Input: part model. Units: mm. Frame: model coordinates. A direction names the side the tool comes from. Give positions to 0.01 mm unless a question says otherwise; leave off trailing zeros. Loops run counter-clockwise (first coordinate to the right, second up) from the corner with the lowest first, then second, coordinate; pieces in that order, holes last. Notation, with made-up numbers: M 51,-5 L 94,-5 A23 cw 94,4 Z; hole C 51.5,-39 d2. An arc over 180 degrees is marked long. Use CSV: the item, a comma, the result in double quotes. Start each with the question number.
Q1. Section C-C, the plane x = -32.55. Output: boundary loops of the cut face in (y, z), plus the area to 3 significant figures.
Q2. Material intervals for line 1 along Y through (x, z) = (-33.45, 17.3); line 2 along Z through (x, y) = (-33.05, -18.75); line 3 along Z through (x, y) = (-32.35, -19.5), sorted ascending.
Q3. Section D-D, the plane z = 2. Output: boundary loops of the cut face in (x, y).
Q4. Pin query (flat end, axial travel): pin 1 (1.3 mm diameter, centred on x = -30.5, y = -29.5, fed in from +Z); pin 2 (3.5 mm diameter, centred on y = -40, z = 17.3, fed in from +X); pin 3 (1.2 mm diameter, centred on x = -32, z = 7, fed in from +Y). Return the tip coordinate at first contact, or that it passes through.
Q5. Pull-direction query (Y, two-part tool) for faces 1 (the flat face through (-33, -29, 20)), 2 (the flat face through (-32, -42.5, 13)), 3 (the cylindrical face through (-30.51, -17.59, 3.04)), 4 (the flat face through (-32, -15.5, 13)); classes: released by +Y, released by -Y, zero draft, split by the parting line, or undercut.
Q6. Section B-B, the plane y = -40. Output: boundary loops of the cut face in (x, z).
Q7. Section A-A, the plane z = 17.3. Output: boundary loops of the cut face in (x, y).
Q8. Reachability of faces 5 (the flat face through (-32, -18, 8.5)), 6 (the cylindrical face through (-32.087, -41.318, 3.042)), 7 (the flat face through (-32, -37.5, 7)) from +Z, -Z, +X, -X, +Y, -Y: full face, straight path, thin tool, end or side. Return the list, or none.
Autodesk Inventor part; units mm, degrees
ref_plane "작업 평면1" through (-17.0116, -44.6019, 14.5) normal (0, 0, -1) x (0, 1, 0)
ref_plane "YZ Plane" through (0, 0, 0) normal (1, 0, 0) x (0, 1, 0)
ref_plane "XZ Plane" through (0, 0, 0) normal (0, 1, 0) x (-1, 0, 0)
ref_plane "작업 평면1" through (-17.0116, -44.6019, 14.5) normal (0, 0, -1) x (0, 1, 0)
sketch "스케치4" plane through (0, 0, 0) normal (0, 0, 1) x (1, 0, 0)
  arc A0 (-34.0751, 6.2636) -> (-34.5943, 4.5766) centre (-31.5943, 4.5766) ccw
  line L0 (-34.5943, -39.6766) -> (-34.5943, 4.5766)
  arc A1 (-34.5943, -39.6766) -> (-34.0751, -41.3636) centre (-31.5943, -39.6766) ccw
  line L1 (-30.3872, -46.7869) -> (-34.0751, -41.3636)
  arc A2 (-30.3872, -46.7869) -> (-27.9064, -48.1) centre (-27.9064, -45.1) ccw
  line L2 (-1.0822, -48.1) -> (-27.9064, -48.1)
  arc A3 (-1.0822, -48.1) -> (1.3986, -46.7869) centre (-1.0822, -45.1) ccw
  line L3 (5.0865, -41.3636) -> (1.3986, -46.7869)
  arc A4 (5.0865, -41.3636) -> (5.6057, -39.6766) centre (2.6057, -39.6766) ccw
  line L4 (5.6057, 4.5766) -> (5.6057, -39.6766)
  arc A5 (5.6057, 4.5766) -> (5.0865, 6.2636) centre (2.6057, 4.5766) ccw
  line L5 (1.1009, 12.1246) -> (5.0865, 6.2636)
  arc A6 (1.1009, 12.1246) -> (-0.5529, 13) centre (-0.5529, 11) ccw
  line L6 (-6.8443, 13) -> (-0.5529, 13)
  arc A7 (-5.3443, 11.5) -> (-6.8443, 13) centre (-6.8443, 11.5) ccw
  line L7 (-5.3443, 11.5) -> (-5.3443, 10)
  arc A8 (-5.3443, 10) -> (-2.9943, 7.65) centre (-2.9943, 10) ccw
  line L8 (-2.9943, 7.65) -> (-0.9943, 7.65)
  arc A9 (0.0057, 6.65) -> (-0.9943, 7.65) centre (-0.9943, 6.65) ccw
  line L9 (0.0057, 6.65) -> (0.0057, -36.15)
  arc A10 (-0.9943, -37.15) -> (0.0057, -36.15) centre (-0.9943, -36.15) ccw
  line L10 (-0.9943, -37.15) -> (-2.9943, -37.15)
  arc A11 (-2.9943, -37.15) -> (-5.3443, -39.5) centre (-2.9943, -39.5) ccw
  line L11 (-5.3443, -39.5) -> (-5.3443, -41.5)
  arc A12 (-6.3443, -42.5) -> (-5.3443, -41.5) centre (-6.3443, -41.5) ccw
  line L12 (-6.3443, -42.5) -> (-22.6443, -42.5)
  arc A13 (-23.6443, -41.5) -> (-22.6443, -42.5) centre (-22.6443, -41.5) ccw
  line L13 (-23.6443, -41.5) -> (-23.6443, -39.5)
  arc A14 (-23.6443, -39.5) -> (-25.9943, -37.15) centre (-25.9943, -39.5) ccw
  line L14 (-25.9943, -37.15) -> (-27.9943, -37.15)
  arc A15 (-28.9943, -36.15) -> (-27.9943, -37.15) centre (-27.9943, -36.15) ccw
  line L15 (-28.9943, -36.15) -> (-28.9943, 6.65)
  arc A16 (-27.9943, 7.65) -> (-28.9943, 6.65) centre (-27.9943, 6.65) ccw
  line L16 (-27.9943, 7.65) -> (-25.9943, 7.65)
  arc A17 (-25.9943, 7.65) -> (-23.6443, 10) centre (-25.9943, 10) ccw
  line L17 (-23.6443, 10) -> (-23.6443, 11.5)
  arc A18 (-22.1443, 13) -> (-23.6443, 11.5) centre (-22.1443, 11.5) ccw
  line L18 (-28.4357, 13) -> (-22.1443, 13)
  arc A19 (-28.4357, 13) -> (-30.0896, 12.1246) centre (-28.4357, 11) ccw
  line L19 (-34.0751, 6.2636) -> (-30.0896, 12.1246)
  circle A20 centre (2.8057, 4) radius 1.35
  circle A21 centre (2.8057, -18) radius 1.35
  circle A22 centre (-3.4943, -45.3) radius 1.35
  circle A23 centre (-31.7943, 4) radius 1.35
  circle A24 centre (-31.7943, -18) radius 1.35
  circle A25 centre (-25.4943, -45.3) radius 1.35
  circle A26 centre (2.8057, -40) radius 1.35
  circle A27 centre (-31.7943, -40) radius 1.35
  line L20 (-31.7943, -40) -> (-31.7943, -18)
  line L21 (-29.0943, -15.5) -> (-34.4943, -15.5)
  line L22 (-34.4943, -15.5) -> (-34.4943, -42.5)
  line L23 (-34.4943, -42.5) -> (-29.0943, -42.5)
  line L24 (-29.0943, -42.5) -> (-29.0943, -15.5)
  line L25 (-29.0943, -15.5) -> (-34.4943, -42.5) construction
  line L26 (-34.4943, -15.5) -> (-29.0943, -42.5) construction
  point P0 (0, 0)
  point P1 (-31.7943, -29)
  dimension "d10" = 5.4
  dimension "d11" = 27
extrude "돌출4" add sketch "스케치4" against normal blind 6 contours L22 L21 L24 L23 L1 A1 | A1 L1 L23 L22
sketch "스케치5" plane through (0, 0, 0) normal (0, 0, 1) x (1, 0, 0)
  line L0 (-34.4943, -15.5) -> (-34.4943, -42.5)
  line L1 (-34.4943, -42.5) -> (-29.0943, -42.5)
  line L2 (-29.0943, -42.5) -> (-29.0943, -15.5)
  line L3 (-29.0943, -15.5) -> (-34.4943, -15.5)
  circle A0 centre (-31.7943, -40) radius 1.35
  circle A1 centre (-31.7943, -18) radius 1.35
  point P0 (0, 0)
extrude "돌출5" add sketch "스케치5" along normal blind 14.4 contours L3 L2 L1 L0 | A0 | A1
sketch "스케치6" plane through (-34.4943, -42.5, -6) normal (-1, 0, 0) x (0, 0, 1)
  line L0 (25.6, 57) -> (29.1, 57)
  line L1 (25.6, 57) -> (20.5, 51)
  line L2 (20.5, 51) -> (20.5, -2.1)
  line L3 (20.5, -2.1) -> (25.6, -8.1)
  line L4 (25.6, -8.1) -> (55.6, -8.1)
  line L5 (55.6, -8.1) -> (60.7, -2.1)
  line L6 (60.7, -2.1) -> (60.7, 51)
  line L7 (60.7, 51) -> (55.6, 57)
  line L8 (52.1, 57) -> (55.6, 57)
  arc A0 (55.1, 54) -> (52.1, 57) centre (52.1, 54) ccw
  line L9 (55.1, 0.5) -> (55.1, 54)
  arc A1 (52.1, -2.5) -> (55.1, 0.5) centre (52.1, 0.5) ccw
  line L10 (29.1, -2.5) -> (52.1, -2.5)
  arc A2 (26.1, 0.5) -> (29.1, -2.5) centre (29.1, 0.5) ccw
  line L11 (26.1, 54) -> (26.1, 0.5)
  arc A3 (29.1, 57) -> (26.1, 54) centre (29.1, 54) ccw
  circle A4 centre (57.9, 46.5) radius 1.35
  circle A5 centre (57.9, 24.5) radius 1.35
  circle A6 centre (57.9, 2.5) radius 1.35
  circle A7 centre (51.6, -5.3) radius 1.35
  circle A8 centre (23.3, 46.5) radius 1.35
  circle A9 centre (23.3, 24.5) radius 1.35
  circle A10 centre (23.3, 2.5) radius 1.35
  circle A11 centre (29.6, -5.3) radius 1.35
  line L12 (20.4, 27) -> (0, 27)
  line L13 (0, 0) -> (0, 27)
  line L14 (0, 0) -> (20.4, 0)
  line L15 (20.4, 27) -> (20.4, 0)
  line L16 (20.4, 0) -> (20.4, 27)
  line L17 (20.4, 27) -> (26, 27)
  line L18 (26, 27) -> (26, 0)
  line L19 (26, 0) -> (20.4, 0)
  line L20 (25.6959, -1.4327) -> (25.7781, -6.0132)
  line L21 (68.9946, 18.9724) -> (67.812, 18.9512)
  arc A12 (65.7765, 20.915) -> (67.812, 18.9512) centre (67.7762, 20.9508) ccw
  line L22 (65.7765, 20.915) -> (65.7397, 22.9646)
  arc A13 (65.7397, 22.9646) -> (64.7219, 23.9465) centre (64.7399, 22.9467) ccw
  line L23 (64.7219, 23.9465) -> (31.7272, 23.3545)
  arc A14 (31.7272, 23.3545) -> (30.7453, 22.3368) centre (31.7452, 22.3547) ccw
  line L24 (30.7453, 22.3368) -> (30.7821, 20.2871)
  arc A15 (28.8183, 18.2515) -> (30.7821, 20.2871) centre (28.7824, 20.2512) ccw
  line L25 (28.8183, 18.2515) -> (26.8186, 18.2157)
  arc A16 (26.8186, 18.2157) -> (25.8367, 17.1979) centre (26.8366, 17.2158) ccw
  line L26 (25.8367, 17.1979) -> (26.0574, 4.8999)
  arc A17 (26.0574, 4.8999) -> (27.0752, 3.918) centre (27.0572, 4.9178) ccw
  line L27 (27.0752, 3.918) -> (29.0748, 3.9538)
  arc A18 (31.1104, 1.99) -> (29.0748, 3.9538) centre (29.1107, 1.9542) ccw
  line L28 (31.1104, 1.99) -> (31.1472, -0.0596)
  arc A19 (31.1472, -0.0596) -> (32.165, -1.0415) centre (32.147, -0.0417) ccw
  line L29 (32.165, -1.0415) -> (65.1596, -0.4495)
  arc A20 (65.1596, -0.4495) -> (66.1415, 0.5682) centre (65.1417, 0.5503) ccw
  line L30 (66.1415, 0.5682) -> (66.1048, 2.6179)
  arc A21 (68.0686, 4.6535) -> (66.1048, 2.6179) centre (68.1044, 2.6538) ccw
  line L31 (68.0686, 4.6535) -> (69.2511, 4.6747)
  spline S0 degree 3 poles (69.2511, 4.6747) (69.5339, 4.6798) (69.869, 4.7337) (70.3387, 4.9133) (70.5662, 5.0474) (70.8526, 5.3129) (70.9739, 5.4731) (71.0515, 5.6305) knots 0 0 0 0 0.420045 0.420045 0.746892 0.746892 1 1 1 1
  line L32 (71.1676, -0.8418) -> (71.0515, 5.6305)
  line L33 (65.2601, -6.0486) -> (71.1676, -0.8418)
  line L34 (26.6663, -6.7411) -> (65.2601, -6.0486)
  line L35 (20.5758, -1.7496) -> (26.6663, -6.7411)
  line L36 (20.1201, 23.6464) -> (20.5758, -1.7496)
  line L37 (26.0277, 28.8532) -> (20.1201, 23.6464)
  line L38 (64.6215, 29.5456) -> (26.0277, 28.8532)
  line L39 (70.712, 24.5541) -> (64.6215, 29.5456)
  line L40 (70.8281, 18.0818) -> (70.712, 24.5541)
  spline S1 degree 3 poles (70.8281, 18.0818) (70.7449, 18.2363) (70.6179, 18.3921) (70.3222, 18.6471) (70.09, 18.7729) (69.6142, 18.9356) (69.2774, 18.9775) (68.9946, 18.9724) knots 0 0 0 0 0.253108 0.253108 0.579955 0.579955 1 1 1 1
  circle A22 centre (63.1719, 26.7192) radius 1.35
  circle A23 centre (46.1747, 26.4142) radius 1.35
  circle A24 centre (22.995, 19.4973) radius 1.35
  circle A25 centre (63.7101, -3.276) radius 1.35
  circle A26 centre (46.7129, -3.581) radius 1.35
  circle A27 centre (23.3, 2.5) radius 1.35
  circle A28 centre (29.1774, 26.1092) radius 1.35
  circle A29 centre (29.7156, -3.8859) radius 1.35
  line L41 (26, 23.5159) -> (0, 23.5159)
  point P0 (6, 42.5)
  dimension "d16" = 5.6
extrude "돌출6" add sketch "스케치6" against normal blind 2.9 contours L17 L37 L2 | L2 L37 L15 L17 | L37 L17 L18 L41 A9 L2 | L2 L41 L15 L37 | L41 A9 L18 A16 L26 L19 L36 L2 | L2 L36 L15 L41 | L18 L26 A16 | L36 L19 L2 | L2 L19 L15 L36 | A24
sketch "스케치7" plane through (-34.4943, -42.5, -6) normal (-1, 0, 0) x (0, 0, 1)
  line L0 (0, 1.15) -> (0, 3.85)
  line L1 (6, 3.85) -> (6, 1.15)
  line L2 (0, 23.15) -> (0, 25.85)
  line L3 (0, 23.15) -> (0, 25.85)
  line L4 (6, 2.5) -> (0, 2.5)
  line L5 (0, 2.5) -> (0, 24.5)
  line L6 (0, 24.5) -> (6, 24.5)
  line L7 (6, 24.5) -> (6, 2.5)
  line L8 (6, 2.5) -> (6, 24.5)
  line L9 (6, 24.5) -> (7.25, 24.5)
  line L10 (7.25, 24.5) -> (7.25, 2.5)
  line L11 (7.25, 2.5) -> (6, 2.5)
  line L12 (8.5, 5) -> (6, 5)
  line L13 (6, 5) -> (6, 0)
  line L14 (6, 0) -> (8.5, 0)
  line L15 (8.5, 0) -> (8.5, 5)
  line L16 (8.5, 5) -> (6, 0) construction
  line L17 (6, 5) -> (8.5, 0) construction
  line L18 (8.5, 22) -> (6, 22)
  line L19 (6, 22) -> (6, 27)
  line L20 (6, 27) -> (8.5, 27)
  line L21 (8.5, 27) -> (8.5, 22)
  line L22 (8.5, 22) -> (6, 27) construction
  line L23 (6, 22) -> (8.5, 27) construction
  point P0 (6, 42.5)
  point P1 (6, 5)
  point P2 (6, 1.15)
  dimension "d19" = 1.25
  dimension "d20" = 2.5
  dimension "d21" = 5
  dimension "d22" = 2.5
  dimension "d23" = 5
extrude "돌출7" cut sketch "스케치7" against normal through all contours L11 L10 L12 L15 L14 L13 L1 | L1 L7 L12 L10 L11 | L9 L10 L18 L7 | L19 L20 L21 L18 L10 L9
move faces "이동1" translate (0, 0, 6) faces at (-29.5959, -25.5425, -6) (-32.6943, -37.5, 1.6667) (-32.6943, -20.5, 0.8333) (-30.8943, -17.1667, 2.5) (-29.5443, -18, 0) (-30.4487, -18.1086, -4) (-30.8943, -15.5, -2) (-30.8943, -39.1667, 2.5) (-29.5443, -40, 0) (-30.4487, -40.1086, -4) (-32.6943, -42.5, -4)
properties part number "Vertical_Connector_CPY"
A:
1,outline,"M -42.5,0 L -41.12,0 L -41.12,6 L -42.5,6 Z; M -42.5,8.5 L -37.5,8.5 L -37.5,6 L -38.88,6 L -38.88,0 L -19.12,0 L -19.12,6 L -20.5,6 L -20.5,8.5 L -15.5,8.5 L -15.5,20 L -42.5,20 Z; M -16.88,0 L -15.5,0 L -15.5,6 L -16.88,6 Z; hole C -40,17.3 d2.7; hole C -18,17.3 d2.7"
1,area,"477 mm^2"
2,line 1,"-42.5 to -41.35, -38.65 to -19.35, -16.65 to -15.5"
2,line 2,"0 to 6, 8.5 to 16.18, 18.42 to 20"
2,line 3,"0 to 6, 8.5 to 20"
3,outline,"M -34.49,-42.5 L -29.09,-42.5 L -29.09,-15.5 L -34.49,-15.5 Z; hole C -31.79,-40 d2.7; hole C -31.79,-18 d2.7"
4,pin 1,"z = 14.4"
4,pin 2,"x = -31.59"
4,pin 3,"y = -20.5"
5,face 1,"zero draft"
5,face 2,"released by -Y"
5,face 3,"undercut"
5,face 4,"released by +Y"
6,outline,"M -34.49,0 L -33.14,0 L -33.14,6 L -34.49,6 Z; M -34.49,8.5 L -29.09,8.5 L -29.09,14.4 L -31.59,14.4 L -31.59,15.95 L -34.49,15.95 Z; M -34.49,18.65 L -31.59,18.65 L -31.59,20 L -34.49,20 Z; M -30.44,0 L -29.09,0 L -29.09,6 L -30.44,6 Z"
7,outline,"M -34.49,-42.5 L -31.59,-42.5 L -31.59,-41.35 L -34.49,-41.35 Z; M -34.49,-38.65 L -31.59,-38.65 L -31.59,-19.35 L -34.49,-19.35 Z; M -34.49,-16.65 L -31.59,-16.65 L -31.59,-15.5 L -34.49,-15.5 Z"
8,face 5,"+X, -X, +Y"
8,face 6,"-Z"
8,face 7,"+X, -X, -Y"
